```python
from build123d import *

# Parameters (mm, degrees)
SKETCH1_W               = 16
SKETCH1_H               = 60
BOSS_EXTRUDE1_DEPTH     = 12
CUT_EXTRUDE1_DEPTH      = 62.708994482
CUT_EXTRUDE1_DEPTH_BACK = 62.708994482
CUT_EXTRUDE3_DEPTH      = 62.708994482
CUT_EXTRUDE3_DEPTH_BACK = 62.708994482
SKETCH4_R               = 3
SKETCH4_R_2             = 1.5
BOSS_EXTRUDE2_DEPTH     = 2.5
FILLET1_R               = 1
CUT_EXTRUDE4_DEPTH      = 62.708994482
FILLET2_R               = 10
SKETCH6_W               = 4.913298596
SKETCH6_H               = 8.315277322
SKETCH6_H_2             = 8.493571251
CUT_EXTRUDE5_DEPTH      = 5
SKETCH7_W               = 4.913298596
SKETCH7_H               = 8.493571251
CUT_EXTRUDE6_DEPTH      = 62.708994482
CUT_EXTRUDE7_REACH      = 44.091
SKETCH8_W               = 4.913298596
SKETCH8_H               = 2.5


with BuildPart() as part:
    # Sketch1 → Boss-Extrude1 (new body)
    with BuildSketch(Plane.XY):
        with Locations((0, -30)):
            Rectangle(SKETCH1_W, SKETCH1_H)
    extrude(amount=BOSS_EXTRUDE1_DEPTH)

    # Sketch2 → Cut-Extrude1 (cut, two sides: drawn at the far end of the back side and taken through both)
    with BuildSketch(Plane(origin=(0, 0, 0), x_dir=(0, 0, -1), z_dir=(1, 0, 0)).offset(-CUT_EXTRUDE1_DEPTH_BACK)):
        Polygon((-8, 0), (0, 0), (0, -8), align=None)
    extrude(amount=CUT_EXTRUDE1_DEPTH + CUT_EXTRUDE1_DEPTH_BACK, mode=Mode.SUBTRACT)

    # Sketch3 → Cut-Extrude3 (cut, two sides: drawn at the far end of the back side and taken through both)
    with BuildSketch(Plane(origin=(0, 0, 0), x_dir=(0, 0, -1), z_dir=(1, 0, 0)).offset(-CUT_EXTRUDE3_DEPTH_BACK)):
        with BuildLine():
            ThreePointArc((-3, 1.1), (-6.559834153, 4.04730143), (-8.791057147, 0))
            Line((-8.791057147, 0), (-7.019803903, 0))
            ThreePointArc((-7.019803903, 0), (-6.600122548, 2.474719218), (-4.5, 1.1))
            ThreePointArc((-4.5, 1.1), (-4.625280782, 0.499877452), (-4.980196097, 0))
            Line((-4.980196097, 0), (-3.208942853, 0))
            ThreePointArc((-3.208942853, 0), (-3.05269857, 0.540165847), (-3, 1.1))
        make_face()
        with BuildLine():
            Line((-7.019803903, 0), (-8.791057147, 0))
            ThreePointArc((-8.791057147, 0), (-6, -1.9), (-3.208942853, 0))
            Line((-3.208942853, 0), (-4.980196097, 0))
            ThreePointArc((-4.980196097, 0), (-6, -0.4), (-7.019803903, 0))
        make_face()
    extrude(amount=CUT_EXTRUDE3_DEPTH + CUT_EXTRUDE3_DEPTH_BACK, mode=Mode.SUBTRACT)

    # Sketch4 → Boss-Extrude2 (add, symmetric)
    with BuildSketch(Plane(origin=(0, 0, 0), x_dir=(0, 0, -1), z_dir=(1, 0, 0))):
        with Locations((-6, 1.1)):
            Circle(SKETCH4_R)
        with Locations((-6, 1.1)):
            Circle(SKETCH4_R_2, mode=Mode.SUBTRACT)
    extrude(amount=BOSS_EXTRUDE2_DEPTH, both=True)

    # Fillet1
    fillet1_edges = [part.edges().sort_by_distance(p)[0] for p in [
        (0, -1.898274836, 6.101725164),
        (0, 0, 8.791057147),
    ]]
    fillet(fillet1_edges, radius=FILLET1_R)

    # Sketch5 → Cut-Extrude4 (cut, through all)
    with BuildSketch(Plane(origin=(0, 0, 0), x_dir=(-1, 0, 0), z_dir=(0, 0, -1))):
        Polygon((0, -60), (8, -22.851648758), (8, -60), align=None)
    extrude(amount=-CUT_EXTRUDE4_DEPTH, mode=Mode.SUBTRACT)

    # Fillet2
    fillet2_edges = [part.edges().sort_by_distance(p)[0] for p in [
        (0, -8, 0),
    ]]
    fillet(fillet2_edges, radius=FILLET2_R)

    # Sketch6 → Cut-Extrude5 (cut)
    with BuildSketch(Plane(origin=(0, 0, 0), x_dir=(-1, 0, 0), z_dir=(0, 0, -1))):
        with Locations((0, -16.299774285)):
            Rectangle(SKETCH6_W, SKETCH6_H)
        with Locations((0, -33.604863133)):
            Rectangle(SKETCH6_W, SKETCH6_H_2)
    extrude(amount=-CUT_EXTRUDE5_DEPTH, mode=Mode.SUBTRACT)

    # Sketch7 → Cut-Extrude6 (cut, through all)
    with BuildSketch(Plane(origin=(0, 0, 0), x_dir=(-1, 0, 0), z_dir=(0, 0, -1))):
        with Locations((0, -33.604863133)):
            Rectangle(SKETCH7_W, SKETCH7_H)
    extrude(amount=-CUT_EXTRUDE6_DEPTH, mode=Mode.SUBTRACT)

    # Sketch8 → Cut-Extrude7 (cut, up to next)
    with BuildSketch(Plane(origin=(0, -20.457412946, 0), x_dir=(1, 0, 0), z_dir=(0, 1, 0)), mode=Mode.PRIVATE) as cut_extrude7_sk1:
        with Locations((0, -3.75)):
            Rectangle(SKETCH8_W, SKETCH8_H)
    cut_extrude7_tool1 = extrude(cut_extrude7_sk1.sketch, amount=-CUT_EXTRUDE7_REACH, mode=Mode.PRIVATE) & part.part
    add(cut_extrude7_tool1.solids().sort_by_distance((0, -20.457413, 3.75))[0], mode=Mode.SUBTRACT)


solid = part.part
```
Input: part model. Units: mm. Frame: model coordinates. A direction names the side the tool comes from. Give positions to 0.01 mm unless a question says otherwise; leave off trailing zeros. Order: outer loops, then holes, each group sorted by start corner. A loop starts at its lowest first (then second) coordinate and runs counter-clockwise, first axis right, second up. Notation, with made-up numbers: (15.5, -19) - (44.5, -19) arc R32 ccw to (44.5, 11) - close; hole circle Ø4 at (6, 17.5). An arc over 180 degrees is marked (long way). Use a Markdown table: item, result.
(1) Access query for faces 1 (the cylindrical face through (5.212, -1.337, 7.75)), 2 (the flat face through (-0.1, 0, 10.4)), 3 (the flat face through (0, -12.142, 2)), 4 (the flat face through (0, -29.358, 8)), 5 (the cylindrical face through (-5.288, -1.337, 7.75)). Directions: +Z, -Z, +X, -X, +Y, -Y. A direction counts if a zero-diameter tool reaches every point of the face in a straight line with its end or side. Return the directions, or none.
Computed values:
| item | result |
|---|---|
| face 1 | -Z, +X, +Y |
| face 2 | +Z, +Y |
| face 3 | -Z |
| face 4 | +Z, -Z |
| face 5 | -Z, -X, +Y |
(2) Section query A-A (x = 7). Output: boundary loops of the cut face in (y, z).
Computed values:
| item | result |
|---|---|
| outline | (-60, 0) - (-12.14, 0) arc R10 ccw to (-5.07, 2.93) - (-1.9, 6.1) arc R3 cw to (0, 8.79) - (0, 12) - (-60, 12) - close |
(3) Section query B-B (x = 1.5). Output: boundary loops of the cut face in (y, z) (3 decimals).
Computed values:
| item | result |
|---|---|
| outline | (-60, 0) - (-37.852, 0) - (-37.852, 12) - (-60, 12) - close; (-29.358, 0) - (-20.457, 0) - (-20.457, 2.5) - (-29.358, 2.5) - close; (-29.358, 5) - (-12.142, 5) - (-12.142, 0) arc R10 ccw to (-5.071, 2.929) - (-3.15, 4.85) arc R1 cw to (-1.557, 4.607) arc R3 ccw (long way) to (1.025, 8.999) arc R1 cw to (0, 9.999) - (0, 12) - (-29.358, 12) - close; hole circle Ø3 at (1.1, 6) |
(4) Pin query (flat end, axial travel): pin 1 (3.5 mm diameter, centred on y = 2, z = 6, fed in from -X); pin 2 (3.5 mm diameter, centred on y = 2, z = 5, fed in from +X); pin 3 (1 mm diameter, centred on x = -1.5, z = 10.5, fed in from +Y). Return the tip coordinate at first contact, or that it passes through.
Computed values:
| item | result |
|---|---|
| pin 1 | stops at x = -2.5 |
| pin 2 | stops at x = 2.5 |
| pin 3 | stops at y = 0 |
(5) Section query D-D (x = -6.5). Output: boundary loops of the cut face in (y, z).
Computed values:
| item | result |
|---|---|
| outline | (-29.82, 0) - (-12.14, 0) arc R10 ccw to (-5.07, 2.93) - (-1.9, 6.1) arc R3 cw to (0, 8.79) - (0, 12) - (-29.82, 12) - close |
(6) Section query C-C (y = -17). Output: boundary loops of the cut face in (x, z), then the cut area to 3 significant figures.
Computed values:
| item | result |
|---|---|
| outline | (-8, 0) - (-2.46, 0) - (-2.46, 5) - (2.46, 5) - (2.46, 0) - (8, 0) - (8, 12) - (-8, 12) - close |
| area | 167 mm2 |
(7) Line query: line 1 (Y direction, x = 1, z = 6); line 2 (Z direction, x = 1, y = -17); line 3 (X direction, y = -30, z = 11.5). Output: solid intervals per line, ascending. Write a range as from..to.
Computed values:
| item | result |
|---|---|
| line 1 | y = -60..-37.85, -29.36..-0.4, 2.6..4.1 |
| line 2 | z = 5..12 |
| line 3 | x = -6.46..-2.46, 2.46..8 |
(8) Draft query along Z for faces 6 (the flat face through (8, -30, 6)), 7 (the flat face through (0, -25, 2.5)), 8 (the flat face through (3, -36, 0)). Return one class per face: released by +Z, released by -Z, zero draft, split by the parting line, or undercut.
Computed values:
| item | result |
|---|---|
| face 6 | zero draft |
| face 7 | undercut |
| face 8 | released by -Z |
